Part model, mm, in its own coordinate system. A direction names the side the tool comes from. Give positions to 0.01 mm unless a question says otherwise; leave off trailing zeros. Write each loop counter-clockwise with the first axis right and the second up, starting at its lowest first coordinate (ties: lowest second). Pieces come first, ordered by that corner, then holes. Notation, with made-up numbers: (-6, -6.5) - (46, -6.5) arc R37 ccw to (46, 31.5) - close; hole circle Ø10 at (66.5, -22). An arc over 180 degrees is marked (long way). Answer as a JSON object with one key per item and string values. Group by question number.
```python
from build123d import *

# Parameters (mm, degrees)
F1_DEPTH = 6.35
F2_R     = 6.3499
F0_R     = 5.08
F3_DEPTH = 6.35
F0_R_2   = 4.826
F4_DEPTH = 6.35
F5_DEPTH = 6.35


# Not quite as in the source:
# - a fillet or chamfer is up to 0.001 mm smaller than in the source, because OpenCascade refuses the exact size


with BuildPart() as f1:
    # F0 (on Front) → F1 (new body, symmetric)
    with BuildSketch(Plane.XZ):
        with BuildLine():
            Line((38.1, 6.35), (-38.1, 6.35))
            ThreePointArc((-38.1, 6.35), (-36.4445407024, 3.3649028089), (-35.871147458, 0))
            ThreePointArc((-35.871147458, 0), (-36.4445407024, -3.3649028089), (-38.1, -6.35))
            Line((-38.1, -6.35), (38.1, -6.35))
            ThreePointArc((38.1, -6.35), (35.871147458, 0), (38.1, 6.35))
        make_face()
    extrude(amount=F1_DEPTH, both=True)

    # F2 (radius 6.35 in the source; OpenCascade refuses exactly that, so slightly less here)
    f2_edges = [f1.edges().sort_by_distance(p)[0] for p in [
        (0, -6.35, 6.35),
        (0, 6.35, 6.35),
        (0, -6.35, -6.35),
        (0, 6.35, -6.35),
    ]]
    fillet(f2_edges, radius=F2_R)

    # F0 (on Front) → F3 (join)
    with BuildSketch(Plane.XZ):
        with BuildLine():
            Line((38.1, -6.35), (38.1, 6.35))
            ThreePointArc((38.1, 6.35), (35.871147458, 0), (38.1, -6.35))
        make_face()
        with BuildLine():
            ThreePointArc((56.191147458, 0), (49.3960502669, 9.5866067556), (38.1, 6.35))
            Line((38.1, 6.35), (38.1, -6.35))
            ThreePointArc((38.1, -6.35), (49.3960502669, -9.5866067556), (56.191147458, 0))
        make_face()
        with Locations((46.031147458, 0)):
            Circle(F0_R, mode=Mode.SUBTRACT)
    extrude(amount=F3_DEPTH)

    # F0 (on Front) → F4 (join)
    with BuildSketch(Plane.XZ):
        with BuildLine():
            Line((-38.1, -6.35), (-38.1, 6.35))
            ThreePointArc((-38.1, 6.35), (-56.191147458, 0), (-38.1, -6.35))
        make_face()
        with Locations((-46.031147458, 0)):
            Circle(F0_R_2, mode=Mode.SUBTRACT)
        with BuildLine():
            ThreePointArc((-35.871147458, 0), (-36.4445407024, 3.3649028089), (-38.1, 6.35))
            Line((-38.1, 6.35), (-38.1, -6.35))
            ThreePointArc((-38.1, -6.35), (-36.4445407024, -3.3649028089), (-35.871147458, 0))
        make_face()
    extrude(amount=-F4_DEPTH)

    # F0 (on Front) → F5 (join, symmetric)
    with BuildSketch(Plane.XZ):
        with Locations((-46.031147458, 0)):
            Circle(F0_R_2)
    extrude(amount=F5_DEPTH, both=True)


solid = f1.part
```
1) Band-saw the part on B-B (z = 1). List the corners of the cut face in (x, y).
2) Drop flat-ended pins along their axis: P1, Ø3, axis at x = 23, y = 4.5, coming from the -Z side; P2, Ø1, axis at x = 28, y = 2, coming from the +Z side; P3, Ø4, axis at x = 8, z = -3, coming from the -Y side. Give the stop position or say it passes through.
3) Band-saw the part on D-D (y = 3.5). List the corners of the cut face in (x, z), plus the area to 3 significant figures.
4) Mould opens along X. For faces 4 (the cylindrical face through (35.87, 2.42, -0.1)), 5 (the cylindrical face through (-0.53, 4.44, 4.54)), 6 (the cylindrical face through (-35.87, -2.51, 0.1)) say: pulls with the +X half, pulls with the -X half, needs draft (parallel to the pull), parting line crosses it, or undercut.
5) Band-saw the part on A-A (y = -4). List the corners of the cut face in (x, z).
6) Which spindle directions (+Z, -Z, +X, -X, +Y, -Y) get a long thin tool onto all of the face, cutting with end or side? Do faces 1 (the flat face through (-41.66, 0, 2.4)), 2 (the cylindrical face through (0.53, 4.44, -4.54)), 3 (the cylindrical face through (-0.53, -4.44, 4.54)). Say none if no direction does.
7) Probe line 1 (X direction, y = -1.25, z = -2.75); line 2 (Y direction, x = -45.5, z = 8.5); line 3 (X direction, y = -5.5, z = -1.75). List the from-to ranges inside material, lowest first.
Verdict:
{
 "1": {"outline": "(-56.14, 0) - (-50.75, 0) - (-50.75, -6.35) - (-41.31, -6.35) - (-41.31, 0) - (-35.92, 0) - (-35.92, -6.27) - (35.92, -6.27) - (35.92, -6.35) - (41.05, -6.35) - (41.05, 0) - (35.92, 0) - (35.92, 6.27) - (-35.92, 6.27) - (-35.92, 6.35) - (-56.14, 6.35) - close; (51.01, -6.35) - (56.14, -6.35) - (56.14, 0) - (51.01, 0) - close"},
 "2": {"P1": "z = -5.6", "P2": "z = 6.17", "P3": "y = -6.27"},
 "3": {"outline": "(-37.36, -5.3) - (37.36, -5.3) arc R10.16 cw to (37.36, 5.3) - (-37.36, 5.3) arc R10.16 ccw (long way) to start", "area": "1,090 mm2"},
 "4": {"face 4": "pulls with the +X half", "face 5": "needs draft", "face 6": "undercut"},
 "5": {"outline": "circle Ø9.65 at (-46.03, 0); (-37.15, -4.93) - (37.15, -4.93) arc R10.16 ccw (long way) to (37.15, 4.93) - (-37.15, 4.93) arc R10.16 cw to start; hole circle Ø10.16 at (46.03, 0)"},
 "6": {"face 1": "-Y", "face 2": "-Z, +X, +Y", "face 3": "+Z, -Y"},
 "7": {"line 1": "-50 to -42.07, -36.25 to 41.76, 50.3 to 55.81", "line 2": "0 to 6.35", "line 3": "-50.53 to -41.53, -36.02 to 41.26, 50.8 to 56.04"}
}
